The listing builds one solid part. Answer for the finished solid, in the listing's coordinates (mm). A direction names the side the tool comes from. Coordinates: 2 decimals unless noted, no trailing zeros. Order: outer loops, then holes, each group sorted by start corner. A loop starts at its lowest first (then second) coordinate and runs counter-clockwise, first axis right, second up. Notation, with made-up numbers: (19.5, 3.25) -> (44.5, 3.25) arc R19 cw to (44.5, 11.25) -> close; hole circle Ø3 at (-3.5, 43). An arc over 180 degrees is marked (long way). Put each result on its own line as item: value. Start each with the question number.
```python
from build123d import *

# Parameters (mm, degrees)
BOSS_EXTRUDE1_DEPTH = 6.35
SKETCH2_R           = 2.54
CUT_EXTRUDE1_DEPTH  = 235.26250767


with BuildPart() as part:
    # Sketch1 → Boss-Extrude1 (new body)
    with BuildSketch(Plane.XY):
        Polygon((0, 0), (0, 50.8), (25.4, 50.8), (25.4, 25.4), (203.2, 25.4), (203.2, 50.8), (228.6, 50.8), (228.6, 0), align=None)
    boss_extrude1 = extrude(amount=BOSS_EXTRUDE1_DEPTH)

    # Sketch2 → Cut-Extrude1 (cut, through all)
    with BuildSketch(Plane.XY.offset(6.35)):
        with Locations((12.7, 38.1)):
            Circle(SKETCH2_R)
        with Locations((12.7, 12.7)):
            Circle(SKETCH2_R)
        with Locations((38.1, 12.7)):
            Circle(SKETCH2_R)
        with Locations((63.5, 12.7)):
            Circle(SKETCH2_R)
        with Locations((88.9, 12.7)):
            Circle(SKETCH2_R)
        with Locations((114.3, 12.7)):
            Circle(SKETCH2_R)
        with Locations((139.7, 12.7)):
            Circle(SKETCH2_R)
        with Locations((165.1, 12.7)):
            Circle(SKETCH2_R)
        with Locations((190.5, 12.7)):
            Circle(SKETCH2_R)
        with Locations((215.9, 12.7)):
            Circle(SKETCH2_R)
        with Locations(Location((215.9, 38.1, 0), (0, 0, 180))):
            Circle(SKETCH2_R)
    cut_extrude1 = extrude(amount=-CUT_EXTRUDE1_DEPTH, mode=Mode.SUBTRACT)

    # Mirror2: Boss-Extrude1, Cut-Extrude1 across plane
    add(boss_extrude1.mirror(Plane(origin=(0, 50.8, 6.35), x_dir=(0, 0, 1), z_dir=(0, -1, 0))))
    add(cut_extrude1.mirror(Plane(origin=(0, 50.8, 6.35), x_dir=(0, 0, 1), z_dir=(0, -1, 0))), mode=Mode.SUBTRACT)


solid = part.part
```
(1) For a pull along X with two mould halves and no side action, classify faces 1 (the flat face through (0, 52, 3)), 2 (the flat face through (116, 101.6, 3)), 3 (the cylindrical face through (192.923, 13.463, 3.219)) as released by +X, released by -X, zero draft, split by the parting line, or undercut.
(2) The part is cut by section B-B on x = 114.3. Determine the outline of the cut face in (y, z), plus the area to 3 significant figures.
(3) The part is cut by section C-C on x = 175.5. Determine the outline of the cut face in (y, z).
(4) The part is cut by section D-D on z = 4. Count the separate pieces of the cut face and the enclosed holes in it, plus the area to 3 significant figures.
(5) A tool of negligible diameter and unlimited length cuts with its end or side. For faces 4 (the flat face through (116, 0, 3)), 5 (the flat face through (203.2, 51, 3)), from which of +Z, -Z, +X, -X, +Y, -Y can it reach the whole face along a straight path? Write none if from no direction.
(6) Find the intervals of material crossed by L1, parallel to Y at x = 12.7, z = 2; L2, parallel to Y at x = 114.3, z = 1.75; L3, parallel to Y at x = 75.5, z = 4, in increasing order.
(7) The part is cut by section A-A on y = 38.1. Determine the outline of the cut face in (x, z).
Worked out:
1. face 1: released by -X
1. face 2: zero draft
1. face 3: undercut
2. outline: (0, 0) -> (10.16, 0) -> (10.16, 6.35) -> (0, 6.35) -> close; (15.24, 0) -> (25.4, 0) -> (25.4, 6.35) -> (15.24, 6.35) -> close; (76.2, 0) -> (86.36, 0) -> (86.36, 6.35) -> (76.2, 6.35) -> close; (91.44, 0) -> (101.6, 0) -> (101.6, 6.35) -> (91.44, 6.35) -> close
2. area: 258 mm2
3. outline: (0, 0) -> (25.4, 0) -> (25.4, 6.35) -> (0, 6.35) -> close; (76.2, 0) -> (101.6, 0) -> (101.6, 6.35) -> (76.2, 6.35) -> close
4. separate pieces: 1
4. enclosed holes: 23
4. area: 13,700 mm2
5. face 4: +Z, -Z, +X, -X, -Y
5. face 5: +Z, -Z
6. L1: 0 to 10.16, 15.24 to 35.56, 40.64 to 60.96, 66.04 to 86.36, 91.44 to 101.6
6. L2: 0 to 10.16, 15.24 to 25.4, 76.2 to 86.36, 91.44 to 101.6
6. L3: 0 to 25.4, 76.2 to 101.6
7. outline: (0, 0) -> (10.16, 0) -> (10.16, 6.35) -> (0, 6.35) -> close; (15.24, 0) -> (25.4, 0) -> (25.4, 6.35) -> (15.24, 6.35) -> close; (203.2, 0) -> (213.36, 0) -> (213.36, 6.35) -> (203.2, 6.35) -> close; (218.44, 0) -> (228.6, 0) -> (228.6, 6.35) -> (218.44, 6.35) -> close
